For this review, use the dimensioned drawing (mm, ordinates from the lowest corner) and the shaded views. Give positions to 0.01 mm unless a question says otherwise; leave off trailing zeros. Write each loop counter-clockwise with the first axis right and the second up, starting at its lowest first coordinate (ties: lowest second). Pieces come first, ordered by that corner, then holes. Notation, with made-up numbers: (75.25, -40) -> (92.25, -40) arc R38 ccw to (92.25, -1) -> close; hole circle Ø3 at (45.25, -33.75). An arc over 180 degrees is marked (long way). Return JSON: item names as keys, results as strings.
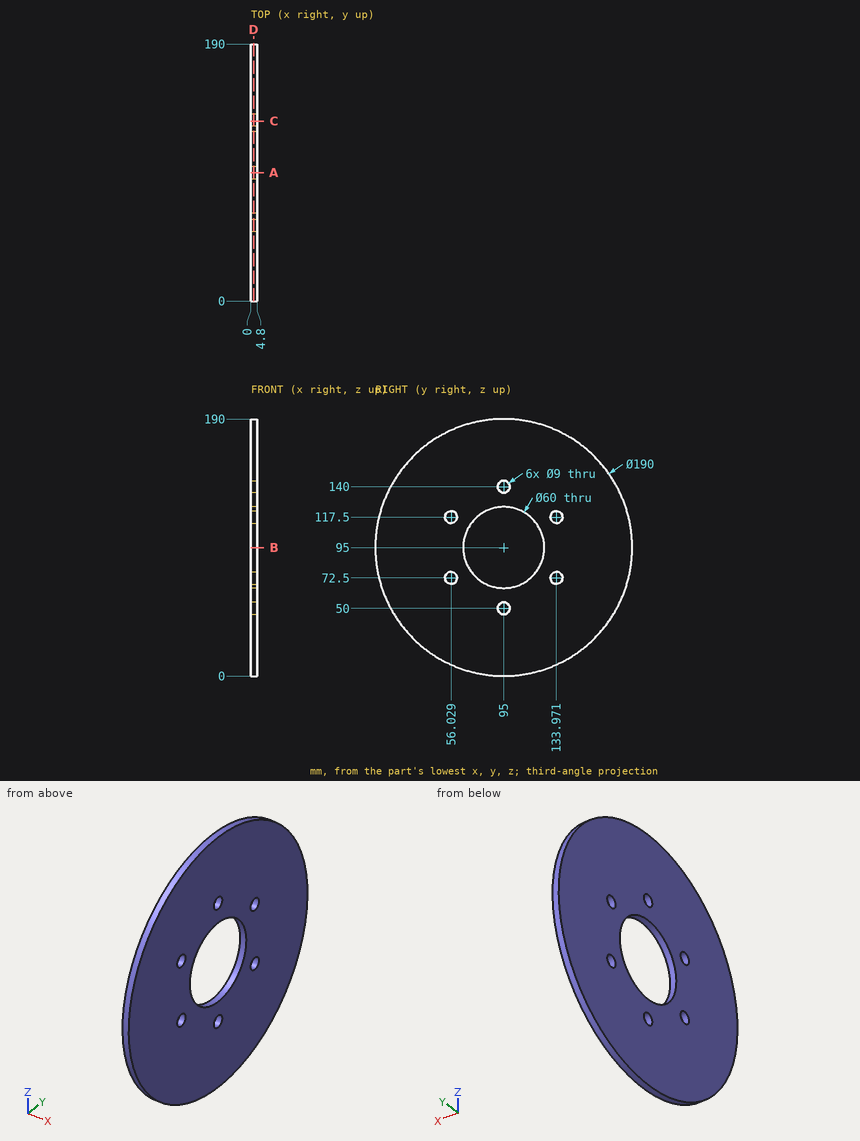
1. Add section D-D, the plane x = 2.2. State the section outline as (y, z) points.
Results found:
{"outline": "circle Ø190 at (95, 95); hole circle Ø9 at (56.03, 72.5); hole circle Ø9 at (56.03, 117.5); hole circle Ø60 at (95, 95); hole circle Ø9 at (95, 50); hole circle Ø9 at (95, 140); hole circle Ø9 at (133.97, 72.5); hole circle Ø9 at (133.97, 117.5)"}
2. Add section A-A, the plane y = 95. State the section outline as (x, z) points, plus the area to 3 significant figures.
Results found:
{"outline": "(0, 0) -> (4.8, 0) -> (4.8, 45.5) -> (0, 45.5) -> close; (0, 54.5) -> (4.8, 54.5) -> (4.8, 65) -> (0, 65) -> close; (0, 125) -> (4.8, 125) -> (4.8, 135.5) -> (0, 135.5) -> close; (0, 144.5) -> (4.8, 144.5) -> (4.8, 190) -> (0, 190) -> close", "area": "538 mm²"}
3. To check wall thickness, follow probe 1 along Z at (x, y) = (1.95, 95); probe 2 along Z at (x, y) = (2.5, 57); probe 3 along Y at (x, z) = (3.2, 95). State the ranges of each line that lie inside material, in increasing order.
Results found:
{"probe 1": "z = 0 to 45.5, 54.5 to 65, 125 to 135.5, 144.5 to 190", "probe 2": "z = 7.93 to 68.11, 76.89 to 113.11, 121.89 to 182.07", "probe 3": "y = 0 to 65, 125 to 190"}
4. Add section B-B, the plane z = 95. State the section outline as (x, y) points, plus the area to 3 significant figures.
Results found:
{"outline": "(0, 0) -> (4.8, 0) -> (4.8, 65) -> (0, 65) -> close; (0, 125) -> (4.8, 125) -> (4.8, 190) -> (0, 190) -> close", "area": "624 mm²"}
5. Add section C-C, the plane y = 133. State the section outline as (x, z) points.
Results found:
{"outline": "(0, 7.93) -> (4.8, 7.93) -> (4.8, 68.11) -> (0, 68.11) -> close; (0, 76.89) -> (4.8, 76.89) -> (4.8, 113.11) -> (0, 113.11) -> close; (0, 121.89) -> (4.8, 121.89) -> (4.8, 182.07) -> (0, 182.07) -> close"}
6. For pin 1 (1.5 mm diameter, centred on x = 3, y = 157, fed in from -Z); pin 2 (1.5 mm diameter, centred on x = 2, z = 161, fed in from -Y); pin 3 (5.5 mm diameter, centred on y = 56.03, z = 117.5, fed in from -X), all flat-tipped, find the tip position at first contact; note any pin that passes through.
Results found:
{"pin 1": "stops at z = 22.38", "pin 2": "stops at y = 25.95", "pin 3": "passes through"}
